Print and shaded views of the part. All mm, measured from the part's lowest x, y and z. A direction names the side the tool comes from. Round coordinates to 2 decimals unless told otherwise and drop trailing zeros. Loops run counter-clockwise (first coordinate to the right, second up) from the corner with the lowest first, then second, coordinate; pieces in that order, holes last. Notation, with made-up numbers: M 61.25,28.5 L 69.25,28.5 A26 ccw 69.25,46.5 Z; hole C 0,89 d3. An arc over 180 degrees is marked long. One line per item, written item: value. Start each with the question number.
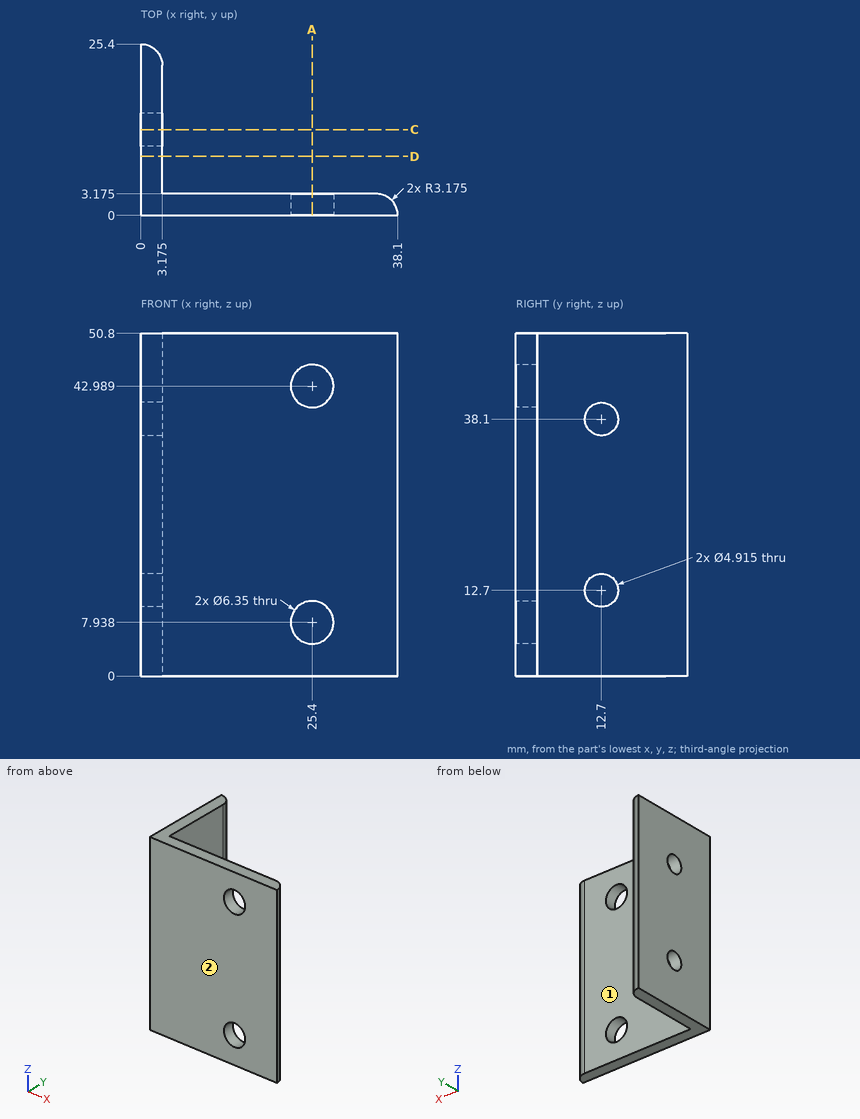
(1) Slice it at C-C, the plane y = 12.7. List the corners of the cut face in (x, z) (1 decimal), and give its area (3 significant figures).
(2) Which spindle directions (+Z, -Z, +X, -X, +Y, -Y) get a long thin tool onto all of the face, cutting with end or side? Do the marked faces 1 and 2. Say none if no direction does.
(3) Flat gauge pins, fed straight in: P1, Ø5, axis at x = 21, z = 13.5, coming from the +Y side (1 decimal); P2, Ø5.5, axis at x = 25.4, z = 7.94, coming from the +Y side; P3, Ø2, axis at y = 15.5, z = 17, coming from the +X side (1 decimal); P4, Ø12, axis at y = 7.5, z = 25.5, coming from the +X side. Where does each tip first touch, or does it go through?
(4) Probe L1, parallel to Z at x = 25.4, y = 2 (1 decimal); L2, parallel to Z at x = 27, y = 3 (1 decimal); L3, parallel to X at y = 16.75, z = 48 (1 decimal). List the from-to ranges inside material, lowest first.
(5) Slice it at D-D, the plane y = 8.75. List the corners of the cut face in (x, z) (1 decimal), and give its area (3 significant figures).
(6) Slice it at A-A, the plane x = 25.4. List the corners of the cut face in (y, z) (1 decimal).
Check result:
1. outline: M 0,0 L 3.2,0 L 3.2,10.2 L 0,10.2 Z; M 0,15.2 L 3.2,15.2 L 3.2,35.6 L 0,35.6 Z; M 0,40.6 L 3.2,40.6 L 3.2,50.8 L 0,50.8 Z
1. area: 130 mm^2
2. face 1: +Z, -Z, +X, +Y
2. face 2: +Z, -Z, +X, -X, -Y
3. P1: stops at y = 3.2
3. P2: passes through
3. P3: stops at x = 3.2
3. P4: stops at x = 37.72
4. L1: z = 0 to 4.8, 11.1 to 39.8, 46.2 to 50.8
4. L2: z = 0 to 5.2, 10.7 to 40.2, 45.7 to 50.8
4. L3: x = 0 to 3.2
5. outline: M 0,0 L 3.2,0 L 3.2,50.8 L 0,50.8 Z
5. area: 161 mm^2
6. outline: M 0,0 L 3.2,0 L 3.2,4.8 L 0,4.8 Z; M 0,11.1 L 3.2,11.1 L 3.2,39.8 L 0,39.8 Z; M 0,46.2 L 3.2,46.2 L 3.2,50.8 L 0,50.8 Z
